Read the model definition and answer for the solid it produces. Units are mm, in the model's axes. A direction names the side the tool comes from. Coordinates: 2 decimals unless noted, no trailing zeros. Write each loop counter-clockwise with the first axis right and the second up, starting at its lowest first coordinate (ties: lowest second). Pieces come first, ordered by that corner, then holes. Notation, with made-up numbers: (-26, -11) - (-15, -11) arc R31 ccw to (-15, 26) - close; hole circle Ø1 at (62, 30.25). An arc over 180 degrees is marked (long way). Return JSON: item names as keys, results as strings.
```python
from build123d import *

# Parameters (mm, degrees)
F0_W     = 130
F0_H     = 5
F0_H_2   = 25
F1_DEPTH = 3
F2_W     = 130
F2_H     = 5
F3_DEPTH = 7
F4_W     = 130
F4_H     = 5
F5_DEPTH = 4
F6_W     = 130
F6_H     = 3
F7_DEPTH = 30


with BuildPart() as f1:
    # F0 (on Top) → F1 (new body)
    with BuildSketch(Plane.XY):
        with Locations((0, 15)):
            Rectangle(F0_W, F0_H)
        Rectangle(F0_W, F0_H_2)
        with Locations((0, -15)):
            Rectangle(F0_W, F0_H)
    extrude(amount=F1_DEPTH)

    # F2 (on face) → F3 (join)
    with BuildSketch(Plane.XY.offset(3)):
        with Locations((0, 15)):
            Rectangle(F2_W, F2_H)
    extrude(amount=F3_DEPTH)

    # F4 (on face) → F5 (join)
    with BuildSketch(Plane.XY.offset(3)):
        with Locations((0, -15)):
            Rectangle(F4_W, F4_H)
    extrude(amount=F5_DEPTH)

    # F6 (on face) → F7 (join)
    with BuildSketch(Plane.XZ.offset(-12.5)):
        with Locations((0, 8.5)):
            Rectangle(F6_W, F6_H)
    extrude(amount=F7_DEPTH)


solid = f1.part
```
(1) Determine the mould class of faces 3 (the face through (-1, 0, 0)), 4 (the face through (-1, 12.5, 5)), 5 (the face through (-1, -17.5, 5)) for opening direction Z: +Z half, -Z half, draft (parallel to the pull), parting line (faces both ways), or undercut.
Answer:
{"face 3": "-Z half", "face 4": "undercut", "face 5": "draft"}
(2) A cutting plane is placed at C-C (y = -3). Determine the outline of the cut face in (x, z).
Answer:
{"outline": "(-65, 0) - (65, 0) - (65, 3) - (-65, 3) - close; (-65, 7) - (65, 7) - (65, 10) - (-65, 10) - close"}
(3) A flat-ended cylindrical pin translates along its axis: P1, Ø3, axis at x = 46.5, y = -0.5, coming from the -Z side. Find the tip coordinate at first contact, or state that the pin passes through.
Answer:
{"P1": "z = 0"}
(4) A cutting plane is placed at A-A (x = 30). Determine the outline of the cut face in (y, z), and give its area (3 significant figures).
Answer:
{"outline": "(-17.5, 0) - (17.5, 0) - (17.5, 10) - (-17.5, 10) - close; hole (-12.5, 3) - (12.5, 3) - (12.5, 7) - (-12.5, 7) - close", "area": "250 mm²"}
(5) Straight lines are drawn through the part: line 1 (Y direction, x = -32, z = 3.5); line 2 (Z direction, x = 39, y = 11). For each, find the intervals that lie inside material, in ascending order. Write a range as from..to.
Answer:
{"line 1": "-17.5..-12.5, 12.5..17.5", "line 2": "0..3, 7..10"}
(6) Which of the six approach directions +Z, -Z, +X, -X, +Y, -Y give full straight-line access (tool end or side, diameter ignored) to faces 1 (the face through (-65, 0.2, 2.7)), 2 (the face through (-1, -12.5, 5))?
Answer:
{"face 1": "+Z, -Z, -X, +Y, -Y", "face 2": "+X, -X"}
(7) A cutting plane is placed at B-B (z = 5.25). Determine the outline of the cut face in (x, y).
Answer:
{"outline": "(-65, -17.5) - (65, -17.5) - (65, -12.5) - (-65, -12.5) - close; (-65, 12.5) - (65, 12.5) - (65, 17.5) - (-65, 17.5) - close"}
